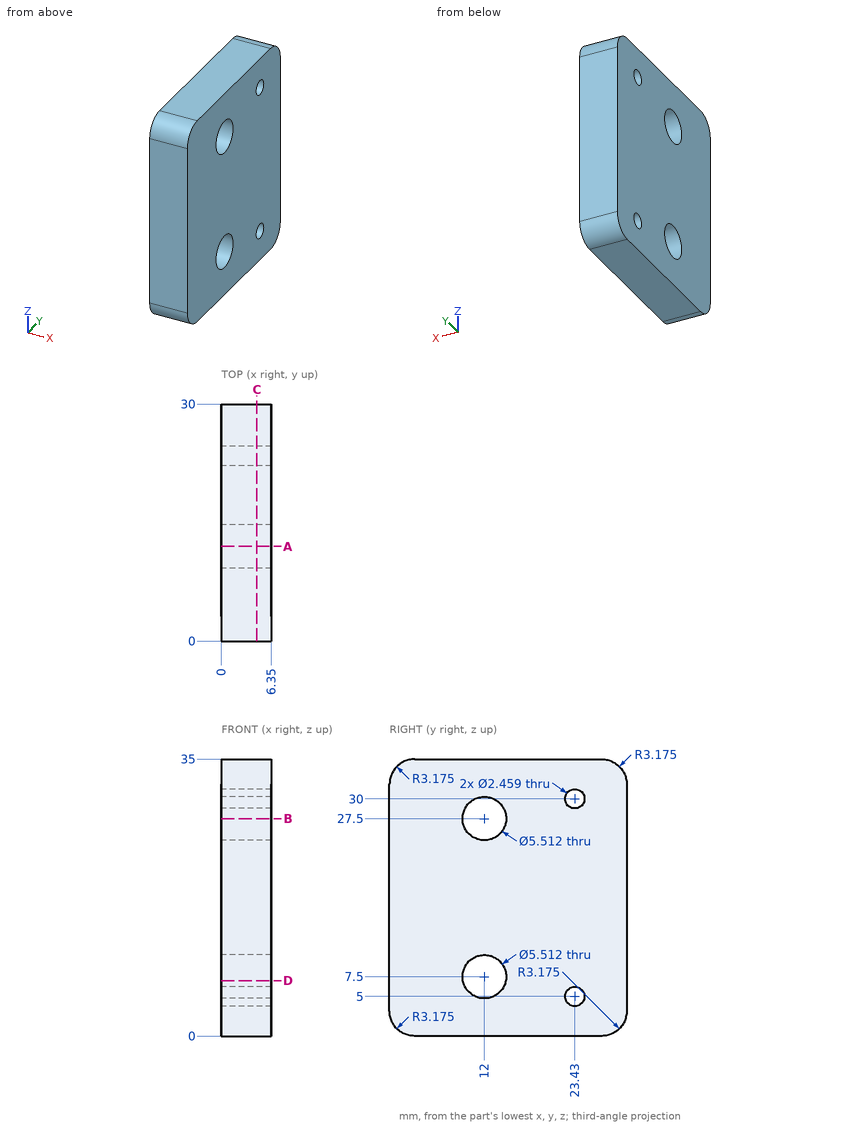
Geometry check sheet. Reference: drawing and pictorial views, mm from the part's lowest x, y, z. Coordinates: 2 decimals unless noted, no trailing zeros. Order: outer loops, then holes, each group sorted by start corner. A loop starts at its lowest first (then second) coordinate and runs counter-clockwise, first axis right, second up.
Item 1: Section check D-D (z = 7). Enter the section's corners in (x, y), plus the area to 3 significant figures.
Item 2: Scan lines: line 1 along Z through (x, y) = (2.5, 23.43); line 2 along Y through (x, z) = (2.25, 27.5); line 3 along Z through (x, y) = (4.75, 12). Record each from-to range of solid material in increasing order.
Item 3: Section check A-A (y = 12). Enter the section's corners in (x, z), plus the area to 3 significant figures.
Item 4: Depth check by flat-ended pin: pin 1 (1.5 mm diameter, centred on y = 23.43, z = 5, fed in from +X). Enter the tip coordinate at first touch or a pass-through.
Item 5: Section check B-B (z = 27.5). Enter the section's corners in (x, y).
Item 6: Section check C-C (x = 4.5). Count the separate pieces of the cut face and the enclosed holes in it, plus the area to 3 significant figures.
Check sheet entries:
1. outline: (0, 0) - (6.35, 0) - (6.35, 9.29) - (0, 9.29) - close; (0, 14.71) - (6.35, 14.71) - (6.35, 30) - (0, 30) - close
1. area: 156 mm2
2. line 1: z = 0 to 3.77, 6.23 to 28.77, 31.23 to 35
2. line 2: y = 0 to 9.24, 14.76 to 30
2. line 3: z = 0 to 4.74, 10.26 to 24.74, 30.26 to 35
3. outline: (0, 0) - (6.35, 0) - (6.35, 4.74) - (0, 4.74) - close; (0, 10.26) - (6.35, 10.26) - (6.35, 24.74) - (0, 24.74) - close; (0, 30.26) - (6.35, 30.26) - (6.35, 35) - (0, 35) - close
3. area: 152 mm2
4. pin 1: passes through
5. outline: (0, 0) - (6.35, 0) - (6.35, 9.24) - (0, 9.24) - close; (0, 14.76) - (6.35, 14.76) - (6.35, 30) - (0, 30) - close
6. separate pieces: 1
6. enclosed holes: 4
6. area: 984 mm2
